Verification items for this drawing (mm, ordinates from the low corner). Give positions to 0.01 mm unless a question says otherwise; leave off trailing zeros. Order: outer loops, then holes, each group sorted by start corner. A loop starts at its lowest first (then second) coordinate and runs counter-clockwise, first axis right, second up. Notation, with made-up numbers: M 56,82.25 L 91,82.25 A16 cw 91,86.25 Z; hole C -7.5,-12.75 d10. An arc over 180 degrees is marked long. Answer as a JSON object with one key per item and string values.
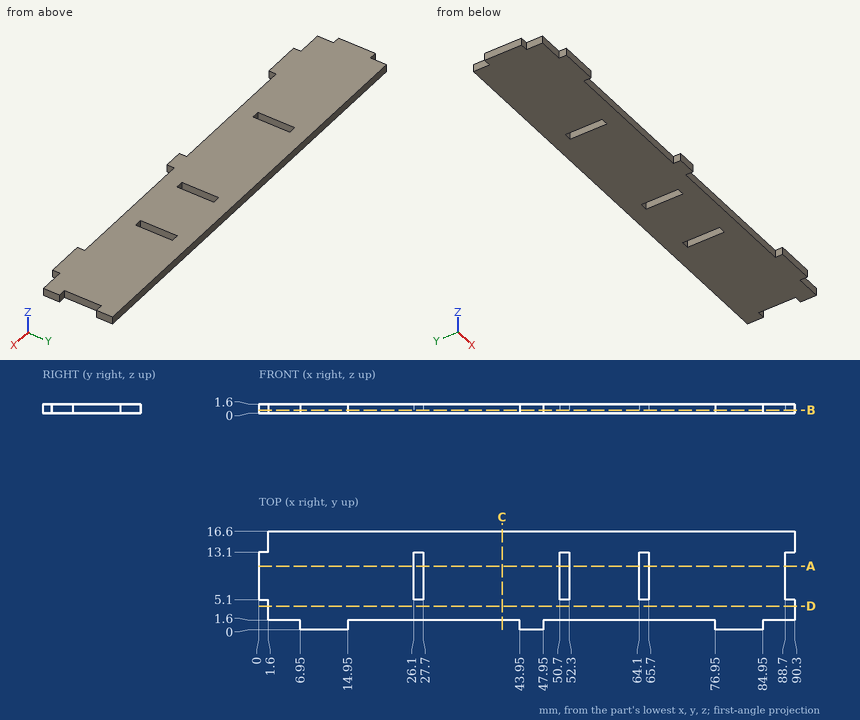
Q1. Material ranges on L1, parallel to X at y = 9.5, z = 0.35; L2, parallel to X at y = 1.25, z = 0.15; L3, parallel to Y at x = 75, z = 1.05, recorded low to high.
Resolved:
{"L1": "x = 0 to 26.1, 27.7 to 50.7, 52.3 to 64.1, 65.7 to 88.7", "L2": "x = 6.95 to 14.95, 43.95 to 47.95, 76.95 to 84.95", "L3": "y = 1.6 to 16.6"}
Q2. Section check D-D on y = 4. Record the cut outline in (x, z).
Resolved:
{"outline": "M 1.6,0 L 90.3,0 L 90.3,1.6 L 1.6,1.6 Z"}
Q3. Section check C-C on x = 41. Record the cut outline in (y, z), then the cut area to 3 significant figures.
Resolved:
{"outline": "M 1.6,0 L 16.6,0 L 16.6,1.6 L 1.6,1.6 Z", "area": "24.0 mm²"}
Q4. Section check A-A on y = 10.75. Record the cut outline in (x, z), then the cut area to 3 significant figures.
Resolved:
{"outline": "M 0,0 L 26.1,0 L 26.1,1.6 L 0,1.6 Z; M 27.7,0 L 50.7,0 L 50.7,1.6 L 27.7,1.6 Z; M 52.3,0 L 64.1,0 L 64.1,1.6 L 52.3,1.6 Z; M 65.7,0 L 88.7,0 L 88.7,1.6 L 65.7,1.6 Z", "area": "134 mm²"}
Q5. Gauge pin test, flat ends, axial feed: pin 1 Ø0.8 at (y, z) = (0.5, 1) entering from -X; pin 2 Ø0.8 at (x, z) = (51.5, 0.5) entering from -Y; pin 3 Ø0.5 at (y, z) = (0.5, 1) entering from +X. Record the tip position at first contact, or that the pin passes through.
Resolved:
{"pin 1": "stops at x = 6.95", "pin 2": "stops at y = 1.6", "pin 3": "stops at x = 84.95"}
Q6. Section check B-B on z = 0.55. Count the separate pieces of the cut face and the enclosed holes in it, then the cut area to 3 significant figures.
Resolved:
{"separate pieces": "1", "enclosed holes": "3", "area": "1,320 mm²"}
